Geometry check sheet. Reference: the model listing, model coordinates, mm. A direction names the side the tool comes from. Coordinates: 2 decimals unless noted, no trailing zeros. Write each loop counter-clockwise with the first axis right and the second up, starting at its lowest first coordinate (ties: lowest second). Pieces come first, ordered by that corner, then holes. Notation, with made-up numbers: (78.5, 69) -> (130.5, 69) arc R35 ccw to (130.5, 101) -> close; hole circle Ø7 at (-17.5, 71). An arc over 180 degrees is marked (long way). Answer in a Markdown table with one row per item. Add a question column.
Q1. Thickness scan on line 1 (X direction, y = 2.7, z = 0); line 2 (Z direction, x = 23, y = 2.7); line 3 (Z direction, x = 22, y = 0.85). Record the ranges inside material, lowest first.
Q2. Section check D-D, the plane y = 2.9. Record the boundary of the cut face in (x, z), and give its area (3 significant figures).
Q3. Section check B-B, the plane z = 0. Record the boundary of the cut face in (x, y), and give its area (3 significant figures).
Q4. Gauge pin test, flat end, axial feed: P1, Ø2, axis at x = 24.5, z = -1, coming from the -Y side. Record the tip position at first contact, or that the pin passes through.
Q5. Section check C-C, the plane x = -21.5. Record the boundary of the cut face in (y, z).
Q6. Section check A-A, the plane y = 0.9. Record the boundary of the cut face in (x, z).
Q7. Tool access check on faces 1 (the face through (0, 4, 0)), 2 (the face through (-25, 1, -3)). Record the directions out of +Z, -Z, +X, -X, +Y, -Y that give a thin tool (end or side, any length) a straight path to the whole face; none if there is none.
```python
from build123d import *

# Parameters (mm, degrees)
SKETCH1_W           = 55
SKETCH1_H           = 12
SKETCH1_R           = 2.25
BOSS_EXTRUDE1_DEPTH = 4
CUT_EXTRUDE1_DEPTH  = 2


with BuildPart() as part:
    # Sketch1 → Boss-Extrude1 (new body)
    with BuildSketch(Plane(origin=(0, 0, 0), x_dir=(1, 0, 0), z_dir=(0, 1, 0))):
        Rectangle(SKETCH1_W, SKETCH1_H)
        with Locations((-23, 0)):
            Circle(SKETCH1_R, mode=Mode.SUBTRACT)
        with Locations((23, 0)):
            Circle(SKETCH1_R, mode=Mode.SUBTRACT)
    extrude(amount=BOSS_EXTRUDE1_DEPTH)

    # Sketch2 → Cut-Extrude1 (cut)
    with BuildSketch(Plane(origin=(0, 0, 0), x_dir=(-1, 0, 0), z_dir=(0, -1, 0))):
        Polygon((-19.449221668, 2.161474783), (-23.096502906, 4.15580163), (-26.647281238, 1.994326847), (-26.550778332, -2.161474783), (-22.903497094, -4.15580163), (-19.352718762, -1.994326847), align=None)
        Polygon((23, 4.156921938), (19.4, 2.078460969), (19.4, -2.078460969), (23, -4.156921938), (26.6, -2.078460969), (26.6, 2.078460969), align=None)
    extrude(amount=-CUT_EXTRUDE1_DEPTH, mode=Mode.SUBTRACT)


solid = part.part
```
Calculated:
| question | item | result |
|---|---|---|
| 1 | line 1 | x = -27.5 to -25.25, -20.75 to 20.75, 25.25 to 27.5 |
| 1 | line 2 | z = -6 to -2.25, 2.25 to 6 |
| 1 | line 3 | z = -6 to -3.56, 3.61 to 6 |
| 2 | outline | (-27.5, -6) -> (27.5, -6) -> (27.5, 6) -> (-27.5, 6) -> close; hole circle Ø4.5 at (-23, 0); hole circle Ø4.5 at (23, 0) |
| 2 | area | 628 mm² |
| 3 | outline | (-27.5, 0) -> (-26.6, 0) -> (-26.6, 2) -> (-25.25, 2) -> (-25.25, 4) -> (-27.5, 4) -> close; (-20.75, 2) -> (-19.4, 2) -> (-19.4, 0) -> (19.4, 0) -> (19.4, 2) -> (20.75, 2) -> (20.75, 4) -> (-20.75, 4) -> close; (25.25, 2) -> (26.6, 2) -> (26.6, 0) -> (27.5, 0) -> (27.5, 4) -> (25.25, 4) -> close |
| 3 | area | 173 mm² |
| 4 | P1 | stops at y = 2 |
| 5 | outline | (0, -6) -> (4, -6) -> (4, -1.68) -> (2, -1.68) -> (2, -3.29) -> (0, -3.29) -> close; (0, 3.29) -> (2, 3.29) -> (2, 1.68) -> (4, 1.68) -> (4, 6) -> (0, 6) -> close |
| 6 | outline | (-27.5, -6) -> (27.5, -6) -> (27.5, 6) -> (-27.5, 6) -> close; hole (-26.6, -2.08) -> (-23, -4.16) -> (-19.4, -2.08) -> (-19.4, 2.08) -> (-23, 4.16) -> (-26.6, 2.08) -> close; hole (19.35, 1.99) -> (19.45, -2.16) -> (23.1, -4.16) -> (26.65, -1.99) -> (26.55, 2.16) -> (22.9, 4.16) -> close |
| 7 | face 1 | +Z, -Z, +X, -X, +Y |
| 7 | face 2 | -Y |
